Verification items for the finished model (mm, model axes). A direction names the side the tool comes from. Give positions to 0.01 mm unless a question says otherwise; leave off trailing zeros. Order: outer loops, then holes, each group sorted by start corner. A loop starts at its lowest first (then second) coordinate and runs counter-clockwise, first axis right, second up.
(1) Gauge pin test, flat ends, axial feed: pin 1 (1.5 mm diameter, centred on x = 16, z = 15.5, fed in from +Y); pin 2 (6 mm diameter, centred on x = 15.5, z = -5.5, fed in from -Y); pin 3 (5 mm diameter, centred on x = 14, z = 9.5, fed in from +Y); pin 4 (12 mm diameter, centred on x = -14, z = -9.5, fed in from +Y). Record the tip position at first contact, or that the pin passes through.
(2) Sectioned sample at A-A on z = -15.5. Record the cut outline in (x, y).
(3) Access from +Z, -Z, +X, -X, +Y, -Y to the whole of each face (thin tool, end or side, straight path). Record for faces 1 (the face through (15, 35, -16)), 2 (the face through (0, 20, 20.5)).
(4) Scan lines: L1, parallel to Z at x = 15.5, y = 38.35; L2, parallel to X at y = 38, z = -15. Record each from-to range of solid material in increasing order.
(5) Sectioned sample at D-D on x = 7. Record the cut outline in (y, z).
(6) Sectioned sample at B-B on y = 10. Record the cut outline in (x, z), plus the area to 3 significant figures.
(7) Sectioned sample at C-C on x = 15.5. Record the cut outline in (y, z).
```python
from build123d import *

# Parameters (mm, degrees)
BOSS_EXTRUDE1_DEPTH = 40
SKETCH2_R           = 11
BOSS_EXTRUDE2_DEPTH = 2
SKETCH3_R           = 2.5
BOSS_EXTRUDE3_DEPTH = 24
SKETCH4_R           = 1.5
CUT_EXTRUDE1_DEPTH  = 5


with BuildPart() as part:
    # Sketch1 → Boss-Extrude1 (new body)
    with BuildSketch(Plane(origin=(0, 0, 0), x_dir=(1, 0, 0), z_dir=(0, 1, 0))):
        Polygon((-16.5, 20.5), (-20.5, 16.5), (-20.5, -16.5), (-16.5, -20.5), (16.5, -20.5), (20.5, -16.5), (20.5, 16.5), (16.5, 20.5), align=None)
    extrude(amount=BOSS_EXTRUDE1_DEPTH)

    # Sketch2 → Boss-Extrude2 (add)
    with BuildSketch(Plane(origin=(0, 40, 0), x_dir=(1, 0, 0), z_dir=(0, 1, 0))):
        Circle(SKETCH2_R)
    extrude(amount=BOSS_EXTRUDE2_DEPTH)

    # Sketch3 → Boss-Extrude3 (add)
    with BuildSketch(Plane(origin=(0, 42, 0), x_dir=(1, 0, 0), z_dir=(0, 1, 0))):
        Circle(SKETCH3_R)
    extrude(amount=BOSS_EXTRUDE3_DEPTH)

    # Sketch4 → Cut-Extrude1 (cut)
    with BuildSketch(Plane(origin=(0, 40, 0), x_dir=(1, 0, 0), z_dir=(0, 1, 0))):
        with Locations((-15.5, 15.5)):
            Circle(SKETCH4_R)
        with Locations((15.5, 15.5)):
            Circle(SKETCH4_R)
        with Locations((15.5, -15.5)):
            Circle(SKETCH4_R)
        with Locations((-15.5, -15.5)):
            Circle(SKETCH4_R)
    extrude(amount=-CUT_EXTRUDE1_DEPTH, mode=Mode.SUBTRACT)


solid = part.part
```
Ans:
1. pin 1: stops at y = 35
1. pin 2: stops at y = 0
1. pin 3: stops at y = 40
1. pin 4: stops at y = 42
2. outline: (-20.5, 0) - (20.5, 0) - (20.5, 40) - (17, 40) - (17, 35) - (14, 35) - (14, 40) - (-14, 40) - (-14, 35) - (-17, 35) - (-17, 40) - (-20.5, 40) - close
3. face 1: +Y
3. face 2: +Z, +X, -X, +Y, -Y
4. L1: z = -20.5 to -17, -14 to 14, 17 to 20.5
4. L2: x = -20.5 to -16.91, -14.09 to 14.09, 16.91 to 20.5
5. outline: (0, -20.5) - (40, -20.5) - (40, -8.49) - (42, -8.49) - (42, 8.49) - (40, 8.49) - (40, 20.5) - (0, 20.5) - close
6. outline: (-20.5, -16.5) - (-16.5, -20.5) - (16.5, -20.5) - (20.5, -16.5) - (20.5, 16.5) - (16.5, 20.5) - (-16.5, 20.5) - (-20.5, 16.5) - close
6. area: 1,650 mm2
7. outline: (0, -20.5) - (40, -20.5) - (40, -17) - (35, -17) - (35, -14) - (40, -14) - (40, 14) - (35, 14) - (35, 17) - (40, 17) - (40, 20.5) - (0, 20.5) - close
